Autodesk Inventor part; units mm, degrees
ref_plane "YZ Plane" through (0, 0, 0) normal (1, 0, 0) x (0, 1, 0)
ref_plane "XZ Plane" through (0, 0, 0) normal (0, 1, 0) x (-1, 0, 0)
ref_plane "XY Plane" through (0, 0, 0) normal (0, 0, 1) x (1, 0, 0)
sketch "Sketch1" plane through (0, 0, 0) normal (0, 1, 0) x (-1, 0, 0)
  line L0 (130, 165) -> (-130, 165)
  line L1 (-130, 165) -> (-130, -165)
  line L2 (-130, -165) -> (130, -165)
  line L3 (130, -165) -> (130, 165)
  point P0 (0, 0)
  point P1 (0, -165)
  point P2 (130, 0)
  dimension "d0" = 260
  dimension "d1" = 330
extrude "Extrusion1" add sketch "Sketch1" along normal blind 100
fillet "Fillet1" radius 5 4 edges at (130, 50, 165) (130, 50, -165) (-130, 50, -165) (-130, 50, 165)
shell "Shell1" thickness 2 removed faces 1 at (43.3333, 100, 53.3333)
sketch "Sketch3" plane through (128, 96, 163) normal (0, 0, -1) x (-1, 0, 0)
  line L0 (251.5, 4) -> (4.5, 4)
  line L1 (138, 4) -> (238, 4)
  line L2 (238, 4) -> (238, -56)
  line L3 (238, -56) -> (138, -56)
  line L4 (138, -56) -> (138, 4)
  line L5 (253, -96) -> (253, 4)
  point P0 (128, -96)
  point P1 (253, 2)
  dimension "d13" = 100
  dimension "d14" = 60
  dimension "d15" = 15
extrude "Extrusion3" add sketch "Sketch3" along normal blind 150
sketch "Sketch4" plane through (-125, 0, 165) normal (0, 0, 1) x (1, 0, 0)
  line L0 (0, 0) -> (0, 100)
  line L1 (0, 0) -> (250, 0)
  line L2 (250, 100) -> (250, 0)
  line L3 (15, 100) -> (115, 100)
  line L4 (15, 40) -> (15, 100)
  line L5 (15, 100) -> (115, 100)
  line L6 (115, 100) -> (115, 40)
  line L7 (115, 40) -> (15, 40)
  line L8 (20, 45) -> (110, 45)
  line L9 (110, 45) -> (110, 109.7523)
  line L10 (110, 109.7523) -> (20, 109.7523)
  line L11 (20, 109.7523) -> (20, 45)
  line L12 (0, 100) -> (250, 100)
  line L13 (0, 100) -> (-3, 100)
  line L14 (-3, 100) -> (0, 100)
  line L15 (0, 100) -> (250, 100)
  line L16 (250, 100) -> (253, 100)
  line L17 (253, 100) -> (250, 100)
  line L18 (250, 100) -> (115, 100)
  line L19 (15, 100) -> (0, 100)
  point P0 (125, 0)
  dimension "d18" = 5
  dimension "d19" = 5
  dimension "d20" = 5
extrude "Extrusion4" cut sketch "Sketch4" against normal blind 150 contours L11 L10 L9 L3 | L3 L9 L8 L11
fillet "Fillet3" radius 5 3 edges at (-60, 45, 165) (-105, 72.5, 165) (-15, 72.5, 165)
sketch "Sketch5" plane through (-125, 0, 165) normal (0, 0, 1) x (1, 0, 0)
  circle A0 centre (235, 85) radius 7.5
  line L0 (115, 100) -> (250, 100)
  line L1 (250, 100) -> (250, 0)
  circle A1 centre (205, 85) radius 7.5
  circle A2 centre (235, 65) radius 7.5
  circle A3 centre (205, 65) radius 7.5
  point P0 (125, 0)
  dimension "d24" = 15
  dimension "d25" = 15
  dimension "d26" = 15
  dimension "d29" = 30
  dimension "d32" = 20
extrude "Extrusion5" add sketch "Sketch5" along normal blind 10
fillet "Fillet4" radius 2 4 edges at (102.5, 85, 175) (102.5, 65, 175) (72.5, 65, 175) (72.5, 85, 175)
sketch "Sketch6" plane through (-125, 0, 165) normal (0, 0, 1) x (1, 0, 0)
  line L0 (120, 95) -> (190, 95)
  line L1 (190, 95) -> (190, 45)
  line L2 (190, 45) -> (120, 45)
  line L3 (120, 45) -> (120, 95)
  line L4 (115, 100) -> (250, 100)
  line L5 (115, 40) -> (115, 100)
  point P0 (125, 0)
  dimension "d38" = 5
  dimension "d39" = 5
  dimension "d40" = 70
  dimension "d41" = 50
extrude "Extrusion6" add sketch "Sketch6" along normal blind 5
chamfer "Chamfer1" distance 2 angle 45 2 edges at (30, 95, 170) (30, 45, 170)
properties part number "case_botten"
Model file for the job. Use its own axes, mm. A direction names the side the tool comes from. Round coordinates to 2 decimals unless told otherwise and drop trailing zeros. Write each loop counter-clockwise with the first axis right and the second up, starting at its lowest first coordinate (ties: lowest second). Pieces come first, ordered by that corner, then holes. Notation, with made-up numbers: (-33.75, 39.25) - (5.25, 39.25) arc R16 ccw to (5.25, 45.25) - close; hole circle Ø2 at (39.25, 60). An arc over 180 degrees is marked (long way). Use CSV: the item, a comma, the result in double quotes. Start each with the question number.
Item 1: Band-saw the part on D-D (x = -52). Write the cut outline in (y, z).
Item 2: Band-saw the part on C-C (z = -109). Write the cut outline in (x, y).
Item 3: Band-saw the part on A-A (z = 20.5). Write the cut outline in (x, y).
Item 4: Pin check, flat tips, straight feed: P1, Ø2.5, axis at x = 38.5, z = 167, coming from the +Y side; P2, Ø2.5, axis at y = 64.5, z = 167.5, coming from the +X side; P3, Ø3, axis at x = 94, z = 50.5, coming from the +Y side; P4, Ø2.5, axis at x = 15.5, z = 166, coming from the -Y side. Stop position of each tip, or through.
Item 5: Tool access for faces 5 (the face through (2, 49, -165)), 6 (the face through (-61, 73, 15)), 7 (the face through (2, 2, 2)), 8 (the face through (117.154, 62.747, 168.944)), 9 (the face through (2, 50, -163)): list every direction of +Z, -Z, +X, -X, +Y, -Y with a clear straight run to the whole face (end or side of a thin tool).
Item 6: Two-plate mould, pull along Z, no slides. Class faces 1 (the face through (74.5, 59.9, 168.9)), 2 (the face through (30, 70, 170)), 3 (the face through (128, 50, 2)), 4 (the face through (-10, 70, 89)): released by +Z, released by -Z, zero draft, split by the parting line, or undercut.
Item 7: Drill centre lines: L1, parallel to X at y = 54, z = 160; L2, parallel to Z at x = -82, y = 76.5; L3, parallel to Y at x = -104, z = 146.5. Where is each one in solid material? Low to high. Write a range as [from, to].
Item 8: Band-saw the part on B-B (x = 110). Write the cut outline in (y, z), and give its area (3 significant figures).
Checked values:
1,outline,"(0, -165) - (100, -165) - (100, -163) - (2, -163) - (2, 163) - (40, 163) - (40, 13) - (100, 13) - (100, 15) - (45, 15) - (45, 160) arc R5 ccw to (40, 165) - (0, 165) - close"
2,outline,"(-130, 0) - (130, 0) - (130, 100) - (128, 100) - (128, 2) - (-128, 2) - (-128, 100) - (-130, 100) - close"
3,outline,"(-130, 0) - (130, 0) - (130, 100) - (128, 100) - (128, 2) - (-128, 2) - (-128, 100) - (-130, 100) - close; (-110, 40) - (-10, 40) - (-10, 100) - (-15, 100) - (-15, 45) - (-105, 45) - (-105, 100) - (-110, 100) - close"
4,P1,"stops at y = 95"
4,P2,"stops at x = 117.5"
4,P3,"stops at y = 2"
4,P4,"stops at y = 0"
5,face 5,"-Z, +X, -X, +Y, -Y"
5,face 6,"+Z, +Y"
5,face 7,"none"
5,face 8,"+Z"
5,face 9,"+Y"
6,face 1,"zero draft"
6,face 2,"released by +Z"
6,face 3,"undercut"
6,face 4,"undercut"
7,L1,"x = [-130, -128], [-110, -105], [-15, -10], [128, 130]"
7,L2,"z = [-165, -163], [13, 15]"
7,L3,"y = [0, 2], [40, 45]"
8,outline,"(0, -165) - (100, -165) - (100, -163) - (2, -163) - (2, 163) - (100, 163) - (100, 165) - (92.5, 165) - (92.5, 173) arc R2 ccw to (90.5, 175) - (79.5, 175) arc R2 ccw to (77.5, 173) - (77.5, 165) - (72.5, 165) - (72.5, 173) arc R2 ccw to (70.5, 175) - (59.5, 175) arc R2 ccw to (57.5, 173) - (57.5, 165) - (0, 165) - close"
8,area,"1,350 mm²"
